from build123d import *

# Parameters (mm, degrees)
SKETCH1_W           = 184.587896
SKETCH1_H           = 35.687
SKETCH1_R           = 2.7039951
SKETCH1_W_2         = 3.429
SKETCH1_H_2         = 8.89
BOSS_EXTRUDE1_DEPTH = 3.302


with BuildPart() as part:
    # Sketch1 → Boss-Extrude1 (new body)
    with BuildSketch(Plane.XY):
        Rectangle(SKETCH1_W, SKETCH1_H)
        with Locations((-86.769448, 0)):
            Circle(SKETCH1_R, mode=Mode.SUBTRACT)
        with Locations((-63.370448, 0)):
            Circle(SKETCH1_R, mode=Mode.SUBTRACT)
        with Locations((63.370448, 0)):
            Circle(SKETCH1_R, mode=Mode.SUBTRACT)
        with Locations((86.769448, 0)):
            Circle(SKETCH1_R, mode=Mode.SUBTRACT)
        with Locations((-86.769448, 9.2075)):
            Rectangle(SKETCH1_W_2, SKETCH1_H_2, mode=Mode.SUBTRACT)
        with Locations((-86.769448, -9.2075)):
            Rectangle(SKETCH1_W_2, SKETCH1_H_2, mode=Mode.SUBTRACT)
        with Locations((-63.370448, 9.2075)):
            Rectangle(SKETCH1_W_2, SKETCH1_H_2, mode=Mode.SUBTRACT)
        with Locations((-63.370448, -9.2075)):
            Rectangle(SKETCH1_W_2, SKETCH1_H_2, mode=Mode.SUBTRACT)
        with Locations((63.370448, -9.2075)):
            Rectangle(SKETCH1_W_2, SKETCH1_H_2, mode=Mode.SUBTRACT)
        with Locations((63.370448, 9.2075)):
            Rectangle(SKETCH1_W_2, SKETCH1_H_2, mode=Mode.SUBTRACT)
        with Locations((86.769448, -9.2075)):
            Rectangle(SKETCH1_W_2, SKETCH1_H_2, mode=Mode.SUBTRACT)
        with Locations((86.769448, 9.2075)):
            Rectangle(SKETCH1_W_2, SKETCH1_H_2, mode=Mode.SUBTRACT)
    extrude(amount=BOSS_EXTRUDE1_DEPTH)


solid = part.part
The model under review builds one solid part; all positions refer to its coordinate system, in mm. Give positions to 0.01 mm unless a question says otherwise; leave off trailing zeros. Order: outer loops, then holes, each group sorted by start corner. A loop starts at its lowest first (then second) coordinate and runs counter-clockwise, first axis right, second up. Notation, with made-up numbers: M -2,-33.5 L 13,-33.5 A18 ccw 13,-26.5 Z; hole C 44,41.5 d10. An arc over 180 degrees is marked long. One line per question, with ' | ' between items. Start each with the question number.
1) Consider section C-C, the plane z = 2.8. State how many separate pieces and enclosed holes the cut face has, then the cut area to 3 significant figures.
2) Consider section A-A, the plane y = 0. Give the boundary of the cut face in (x, z), then the cut area to 3 significant figures.
3) Consider section B-B, the plane x = 63.5. Give the boundary of the cut face in (y, z).
4) Wall thickness on L1, parallel to X at y = 8.5, z = 0.6: over which ranges is the line inside the solid? List them lowest first. Write a range as from..to.
5) Mouldability with a two-part tool opening along X and no side actions: class faces 1 (the face through (61.225, -1.645, 1.628)), 2 (the face through (92.294, 0, 2)) as pulls with the +X half, pulls with the -X half, needs draft (parallel to the pull), parting line crosses it, or undercut.
Found:
1) separate pieces: 1 | enclosed holes: 12 | area: 6,250 mm²
2) outline: M -92.29,0 L -89.47,0 L -89.47,3.3 L -92.29,3.3 Z; M -84.07,0 L -66.07,0 L -66.07,3.3 L -84.07,3.3 Z; M -60.67,0 L 60.67,0 L 60.67,3.3 L -60.67,3.3 Z; M 66.07,0 L 84.07,0 L 84.07,3.3 L 66.07,3.3 Z; M 89.47,0 L 92.29,0 L 92.29,3.3 L 89.47,3.3 Z | area: 538 mm²
3) outline: M -17.84,0 L -13.65,0 L -13.65,3.3 L -17.84,3.3 Z; M -4.76,0 L -2.7,0 L -2.7,3.3 L -4.76,3.3 Z; M 2.7,0 L 4.76,0 L 4.76,3.3 L 2.7,3.3 Z; M 13.65,0 L 17.84,0 L 17.84,3.3 L 13.65,3.3 Z
4) L1: x = -92.29..-88.48, -85.05..-65.08, -61.66..61.66, 65.08..85.05, 88.48..92.29
5) face 1: undercut | face 2: pulls with the +X half
